Geometry: final body of the model. Coordinates: model frame, mm. Face numbers are marked on the shaded views. A direction names the side the tool comes from. Coordinates: 2 decimals unless noted, no trailing zeros. Write each loop counter-clockwise with the first axis right and the second up, starting at its lowest first coordinate (ties: lowest second). Pieces come first, ordered by that corner, then holes. Notation, with made-up numbers: M 28.25,-11.5 L 45.25,-11.5 A30 cw 45.25,17.5 Z; hole C 14,81.25 d8. An arc over 180 degrees is marked long. Write item = value, one per line. Start each with the question number.
Item 1: Section A-A on x = 72. Output: boundary loops of the cut face in (y, z) (3 decimals), plus the area to 3 significant figures.
Item 2: Section B-B on y = 43. Output: boundary loops of the cut face in (x, z) (3 decimals), plus the area to 3 significant figures.
Item 3: First-contact query: pin 1 Ø4 at (x, z) = (80, 56) entering from -Y; pin 2 Ø16.5 at (x, y) = (-7.5, -48.5) entering from +Z (3 decimals); pin 3 Ø8 at (x, y) = (62, 19) entering from +Z; pin 4 Ø19 at (y, z) = (-20.5, 18) entering from -X (3 decimals). Flat tips, straight axial feed; report the tip coordinate or a pass-through.
Item 4: Ray query, L1, parallel to Z at x = 3.5, y = -23 (3 decimals); L2, parallel to X at y = 16, z = 19 (3 decimals); L3, parallel to X at y = -26, z = -1 (3 decimals). Return the intervals inside material, ascending. Write a range as [from, to].
Item 5: Section C-C on z = 4. Output: boundary loops of the cut face in (x, y) (3 decimals).
Item 6: Pull-direction query (X, two-part tool) for the marked faces 5, 6 and 7; classes: +X half, -X half, draft (parallel to the pull), parting line (faces both ways), or undercut.
Item 7: Reachability of the marked faces 1, 2, 3 and 4 from +Z, -Z, +X, -X, +Y, -Y: full face, straight path, thin tool, end or side. Return the list, or none.
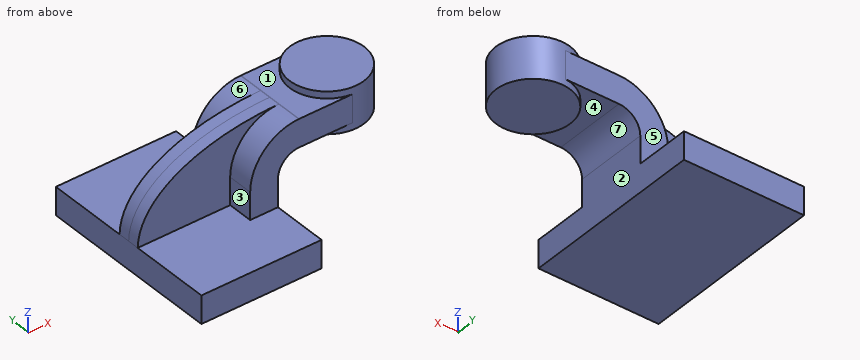
from build123d import *

# Parameters (mm, degrees)
F1_DEPTH = 63.5
F0_W     = 25.2874664307
F0_H     = 19.05
F2_DEPTH = 25.4
F3_DEPTH = 7.9375


with BuildPart() as f1:
    # F0 (on Front) → F1 (new body, symmetric)
    with BuildSketch(Plane.XZ):
        Polygon((-41.275, -9.525), (41.275, -9.525), (41.275, 9.525), (22.225, 9.525), (-41.275, 9.525), align=None)
    extrude(amount=F1_DEPTH, both=True)

    # F0 (on Front) → F2 (join, symmetric)
    with BuildSketch(Plane.XZ):
        with BuildLine():
            Line((22.225, 9.525), (41.275, 9.525))
            Line((41.275, 9.525), (41.275, 28.2031249513))
            ThreePointArc((41.275, 28.2031249513), (45.5723512877, 38.5778487123), (55.9470750487, 42.8752))
            Line((55.9470750487, 42.8752), (69.6396806002, 42.8752))
            Line((69.6396806002, 42.8752), (69.6396806002, 61.9252))
            Line((69.6396806002, 61.9252), (55.9470750487, 61.9252))
            add(Edge.make_bspline(
                [(55.5211131367, 61.9225096141), (55.6629873097, 61.9235358416), (55.8049747134, 61.9244326984), (55.9470750487, 61.9252)],
                knots=[110.1714046274, 110.1714046274, 110.1714046274, 110.1714046274, 110.4441616239, 110.4441616239, 110.4441616239, 110.4441616239], degree=3))
            ThreePointArc((55.5211131367, 61.9225096141), (31.9518394262, 51.8971540095), (22.225, 28.2031249513))
            Line((22.225, 28.2031249513), (22.225, 9.525))
        make_face()
        with Locations((82.2834138155, 52.4002)):
            Rectangle(F0_W, F0_H)
    extrude(amount=F2_DEPTH, both=True)

    # F0 (on Front) → F3 (join, symmetric)
    with BuildSketch(Plane.XZ):
        with BuildLine():
            add(Edge.make_bspline(
                [(-41.275, 9.525), (-40.6163622331, 39.9867175864), (-1.7843899966, 61.50799807), (55.5211131367, 61.9225096141)],
                knots=[0, 0, 0, 0, 110.1714046274, 110.1714046274, 110.1714046274, 110.1714046274], degree=3))
            Line((-41.275, 9.525), (22.225, 9.525))
            Line((22.225, 9.525), (22.225, 28.2031249513))
            ThreePointArc((22.225, 28.2031249513), (31.9518394262, 51.8971540095), (55.5211131367, 61.9225096141))
        make_face()
    extrude(amount=F3_DEPTH, both=True)

    # F0 (on Front) → F4 (revolve)
    with BuildSketch(Plane.XZ):
        Polygon((94.9271470308, 61.9252), (94.9271470308, 42.8752), (94.9271470308, 38.1), (120.4396806002, 38.1), (120.4396806002, 66.675), (94.9271470308, 66.675), align=None)
    revolve(axis=Axis((94.9271470308, 0, 52.3875), (0, 0, -1)))


solid = f1.part
Responses:
q1.outline = M -25.4,42.875 L -11.191,42.875 L -11.191,38.1 L 11.191,38.1 L 11.191,42.875 L 25.4,42.875 L 25.4,61.925 L 11.191,61.925 L 11.191,66.675 L -11.191,66.675 L -11.191,61.925 L -25.4,61.925 Z
q1.area = 1,180 mm²
q2.outline = M -41.275,-9.525 L 41.275,-9.525 L 41.275,9.525 L -41.275,9.525 Z
q2.area = 1,570 mm²
q3.pin_1 = -25.4
q3.pin_2 = 9.525
q3.pin_3 = 61.93
q3.pin_4 = -41.275
q4.L1 = [-9.525, 9.525]
q4.L2 = [22.225, 41.275]
q4.L3 = [-41.275, 41.275]
q5.outline = M -41.275,-63.5 L 41.275,-63.5 L 41.275,63.5 L -41.275,63.5 Z
q6.face_5 = draft
q6.face_6 = -X half
q6.face_7 = undercut
q7.face_1 = +Z, -X
q7.face_2 = -Z, +X, +Y, -Y
q7.face_3 = +Z, -X, -Y
q7.face_4 = -Z
